from build123d import *

# Parameters (mm, degrees)
CYLINDER004_R           = 1.5
CYLINDER004_DEPTH       = 4
CYLINDER005_R           = 1.5
CYLINDER005_DEPTH       = 4
CYLINDER006_R           = 1.5
CYLINDER006_DEPTH       = 4
CYLINDER002_R           = 1.25
CYLINDER002_DEPTH       = 10
CYLINDER002_PITCH_ANGLE = 90
CYLINDER001_R           = 1.55
CYLINDER001_DEPTH       = 50.8
CYLINDER001_PITCH_ANGLE = 90
CYLINDER003_R           = 6
CYLINDER003_DEPTH       = 8
CYLINDER003_PITCH_ANGLE = 90
BOX005_W                = 12
BOX005_H                = 18
BOX005_DEPTH            = 3
BOX004_W                = 8
BOX004_H                = 50
BOX004_DEPTH            = 2.5
BOX003_W                = 12
BOX003_H                = 37
BOX003_DEPTH            = 10
BOX002_W                = 0.4
BOX002_H                = 1
BOX002_DEPTH            = 10
BOX001_W                = 50.8
BOX001_H                = 10
BOX001_DEPTH            = 2
CYLINDER_R              = 5
CYLINDER_DEPTH          = 50.8
CYLINDER_PITCH_ANGLE    = 90
BOX_W                   = 50.8
BOX_H                   = 42
BOX_DEPTH               = 3


with BuildPart() as cylinder004:
    # Cylinder004 → Cylinder004 (new body)
    with BuildSketch(Plane(origin=(12, 10, 3), x_dir=(1, 0, 0), z_dir=(0, 0, 1))):
        Circle(CYLINDER004_R)
    extrude(amount=CYLINDER004_DEPTH)


with BuildPart() as cylinder005:
    # Cylinder005 → Cylinder005 (new body)
    with BuildSketch(Plane(origin=(24, 10, 3), x_dir=(1, 0, 0), z_dir=(0, 0, 1))):
        Circle(CYLINDER005_R)
    extrude(amount=CYLINDER005_DEPTH)


with BuildPart() as cylinder006:
    # Cylinder006 → Cylinder006 (new body)
    with BuildSketch(Plane(origin=(36, 10, 3), x_dir=(1, 0, 0), z_dir=(0, 0, 1))):
        Circle(CYLINDER006_R)
    extrude(amount=CYLINDER006_DEPTH)


with BuildPart() as cylinder002:
    # Cylinder002 → Cylinder002 (new body)
    with BuildSketch(Plane.XY):
        Circle(CYLINDER002_R)
    extrude(amount=CYLINDER002_DEPTH)


with BuildPart() as cylinder002_1:
    # Cylinder002 pitch: moved
    add(cylinder002.part.rotate(Axis((0, 0, 0), (0, 1, 0)), CYLINDER002_PITCH_ANGLE))


with BuildPart() as cylinder002_2:
    # Cylinder002 placement: moved
    add(cylinder002_1.part.moved(Location((-1, 5, -2))))


with BuildPart() as cylinder001:
    # Cylinder001 → Cylinder001 (new body)
    with BuildSketch(Plane.XY):
        Circle(CYLINDER001_R)
    extrude(amount=CYLINDER001_DEPTH)


with BuildPart() as cylinder001_1:
    # Cylinder001 pitch: moved
    add(cylinder001.part.rotate(Axis((0, 0, 0), (0, 1, 0)), CYLINDER001_PITCH_ANGLE))


with BuildPart() as cylinder001_2:
    # Cylinder001 placement: moved
    add(cylinder001_1.part.moved(Location((3, 5, -2))))


with BuildPart() as cylinder003:
    # Cylinder003 → Cylinder003 (new body)
    with BuildSketch(Plane.XY):
        Circle(CYLINDER003_R)
    extrude(amount=CYLINDER003_DEPTH)


with BuildPart() as cylinder003_1:
    # Cylinder003 pitch: moved
    add(cylinder003.part.rotate(Axis((0, 0, 0), (0, 1, 0)), CYLINDER003_PITCH_ANGLE))


with BuildPart() as cylinder003_2:
    # Cylinder003 placement: moved
    add(cylinder003_1.part.moved(Location((24, 5, -2))))


with BuildPart() as cube005:
    # Box005 → Box005 (new body)
    with BuildSketch(Plane(origin=(22, 25, -7), x_dir=(1, 0, 0), z_dir=(0, 0, 1))):
        with Locations((6, 9)):
            Rectangle(BOX005_W, BOX005_H)
    extrude(amount=BOX005_DEPTH)


with BuildPart() as cube004:
    # Box004 → Box004 (new body)
    with BuildSketch(Plane(origin=(24, 10, -4.5), x_dir=(1, 0, 0), z_dir=(0, 0, 1))):
        with Locations((4, 25)):
            Rectangle(BOX004_W, BOX004_H)
    extrude(amount=BOX004_DEPTH)


with BuildPart() as cut002:
    # Box003 → Box003 (new body)
    with BuildSketch(Plane(origin=(22, 5, -7), x_dir=(1, 0, 0), z_dir=(0, 0, 1))):
        with Locations((6, 18.5)):
            Rectangle(BOX003_W, BOX003_H)
    extrude(amount=BOX003_DEPTH)

    # Cut: cut Cube004
    add(cube004.part, mode=Mode.SUBTRACT)

    # Cut001: cut Cube005
    add(cube005.part, mode=Mode.SUBTRACT)

    # Cut002: cut Cylinder003
    add(cylinder003_2.part, mode=Mode.SUBTRACT)


with BuildPart() as cube002:
    # Box002 → Box002 (new body)
    with BuildSketch(Plane(origin=(-0.4, 4.5, -7), x_dir=(1, 0, 0), z_dir=(0, 0, 1))):
        with Locations((0.2, 0.5)):
            Rectangle(BOX002_W, BOX002_H)
    extrude(amount=BOX002_DEPTH)


with BuildPart() as cube001:
    # Box001 → Box001 (new body)
    with BuildSketch(Plane.XY.offset(-2)):
        with Locations((25.4, 5)):
            Rectangle(BOX001_W, BOX001_H)
    extrude(amount=BOX001_DEPTH)


with BuildPart() as cylinder:
    # Cylinder → Cylinder (new body)
    with BuildSketch(Plane.XY):
        Circle(CYLINDER_R)
    extrude(amount=CYLINDER_DEPTH)


with BuildPart() as cylinder_1:
    # Cylinder pitch: moved
    add(cylinder.part.rotate(Axis((0, 0, 0), (0, 1, 0)), CYLINDER_PITCH_ANGLE))


with BuildPart() as cylinder_2:
    # Cylinder placement: moved
    add(cylinder_1.part.moved(Location((0, 5, -2))))


with BuildPart() as fusion003:
    # Box → Box (new body)
    with BuildSketch(Plane.XY):
        with Locations((25.4, 21)):
            Rectangle(BOX_W, BOX_H)
    extrude(amount=BOX_DEPTH)

    # Fusion: union Cube001, Cylinder
    add(cube001.part)
    add(cylinder_2.part)

    # Fusion001: union Cube002
    add(cube002.part)

    # Fusion002: union Cut002
    add(cut002.part)

    # Cut003: cut Cylinder001
    add(cylinder001_2.part, mode=Mode.SUBTRACT)

    # Cut004: cut Cylinder002
    add(cylinder002_2.part, mode=Mode.SUBTRACT)

    # Fusion003: union Cylinder004, Cylinder005, Cylinder006
    add(cylinder004.part)
    add(cylinder005.part)
    add(cylinder006.part)


solid = fusion003.part
Verification items for the finished model (mm, model axes). A direction names the side the tool comes from. Coordinates: 2 decimals unless noted, no trailing zeros. Order: outer loops, then holes, each group sorted by start corner. A loop starts at its lowest first (then second) coordinate and runs counter-clockwise, first axis right, second up. Notation, with made-up numbers: M -24.75,80 L -2.75,80 A12 cw -2.75,86 Z; hole C -20,71.25 d7. An arc over 180 degrees is marked long. Return JSON: item names as keys, results as strings.
1) Access from +Z, -Z, +X, -X, +Y, -Y to the whole of each face (thin tool, end or side, straight path). Record for faces 1 (the flat face through (22, 23, -3)), 2 (the flat face through (34, 23, -3)), 3 (the flat face through (28, 10, -1)), 4 (the flat face through (28, 25, -6)), 5 (the cylindrical face through (10.8, 9.1, 5)).
Answer list:
{"face 1": "-Z, -X, +Y", "face 2": "-Z, +X, +Y", "face 3": "none", "face 4": "-Z, +X, -X, +Y", "face 5": "+Z"}
2) Cross-section at B-B, the plane y = 13. Record the boundary of the cut face in (x, z), and give its area (3 significant figures).
Answer list:
{"outline": "M 0,0 L 22,0 L 22,-7 L 34,-7 L 34,0 L 50.8,0 L 50.8,3 L 0,3 Z; hole M 24,-4.5 L 32,-4.5 L 32,-2 L 24,-2 Z", "area": "216 mm2"}
3) Gauge pin test, flat ends, axial feed: pin 1 (1.5 mm diameter, centred on x = 21.5, y = 23.5, fed in from +Z); pin 2 (1.5 mm diameter, centred on y = 5, z = -2, fed in from -X); pin 3 (8.5 mm diameter, centred on x = 41.5, y = 28.5, fed in from -Z); pin 4 (1.6 mm diameter, centred on x = 6.5, z = -1.5, fed in from +Y). Record the tip position at first contact, or that the pin passes through.
Answer list:
{"pin 1": "z = 3", "pin 2": "through", "pin 3": "z = 0", "pin 4": "y = 10"}
4) Cross-section at C-C, the plane z = 5.25. Record the boundary of the cut face in (x, y), and give its area (3 significant figures).
Answer list:
{"outline": "C 12,10 d3; C 24,10 d3; C 36,10 d3", "area": "21.2 mm2"}
5) Thickness scan on L1, parallel to Y at x = 2.1, z = -2; L2, parallel to Y at x = 15.5, z = -2; L3, parallel to X at y = 9, z = 5.25. Record the ranges inside material, lowest first. Write a range as [from, to].
Answer list:
{"L1": "[0, 3.75], [6.25, 10]", "L2": "[0, 3.45], [6.55, 10]", "L3": "[10.88, 13.12], [22.88, 25.12], [34.88, 37.12]"}
6) Release check for a two-part mould opening along Z. For faces 6 (the flat face through (0, 19.9, 0.3)), 7 (the flat face through (12, 10, 7)), 8 (the cylindrical face through (27.944, 10.916, -0.999)) record: +Z half, -Z half, draft (parallel to the pull), parting line (faces both ways), or undercut.
Answer list:
{"face 6": "draft", "face 7": "+Z half", "face 8": "undercut"}
7) Cross-section at A-A, the plane x = 12. Record the boundary of the cut face in (y, z).
Answer list:
{"outline": "M 0,-2 A5 ccw 10,-2 L 10,0 L 42,0 L 42,3 L 11.5,3 L 11.5,7 L 8.5,7 L 8.5,3 L 0,3 Z; hole C 5,-2 d3.1"}
8) Cross-section at D-D, the plane y = 36.5. Record the boundary of the cut face in (x, z), and give its area (3 significant figures).
Answer list:
{"outline": "M 0,0 L 22,0 L 22,-4 L 24,-4 L 24,-2 L 32,-2 L 32,-4 L 34,-4 L 34,0 L 50.8,0 L 50.8,3 L 0,3 Z", "area": "184 mm2"}
